Work out the finished part from the listing and answer in its coordinate system (mm). Face numbers are marked on the shaded views. A direction names the side the tool comes from. Coordinates: 2 decimals unless noted, no trailing zeros. Order: outer loops, then holes, each group sorted by start corner. A loop starts at its lowest first (then second) coordinate and runs counter-clockwise, first axis right, second up. Notation, with made-up numbers: M -21.75,51 L 18.25,51 A12 cw 18.25,55 Z; hole C 62,86.25 d10. An arc over 180 degrees is marked long. Write item = value, one per line. Start each with the question number.
Q1. Straight lines are drawn through the part: line 1 along Y through (x, z) = (1.25, 13); line 2 along Z through (x, y) = (0.25, -3); line 3 along X through (y, z) = (-1, 19). For each, find the intervals that lie inside material, in ascending order.
Q2. A tool of negligible diameter and unlimited length cuts with its end or side. For the marked faces 1, 2 and 3, from which of +Z, -Z, +X, -X, +Y, -Y can it reach the whole face along a straight path? Write none if from no direction.
Q3. Find section B-B on x = 2.5. Give the vertices of the cut face in (y, z).
Q4. Find section C-C on z = 11. Give the vertices of the cut face in (x, y).
Q5. Find section A-A on y = 1.5. Give the vertices of the cut face in (x, z), and give its area (3 significant figures).
Q6. Each of these flat-tipped pins is pushed along its axis until it touches: P1, Ø1.5, axis at x = 2.5, z = 14.5, coming from the +Y side; P2, Ø1.2, axis at y = 0, z = 16.5, coming from the +X side; P3, Ø3, axis at y = -1, z = 17.5, coming from the -X side; P4, Ø5, axis at x = 1, y = 1.5, coming from the -Z side. Where does it stop, or does it pass through?
Q7. Find section D-D on y = -3.25. Give the vertices of the cut face in (x, z), and give its area (3 significant figures).
Autodesk Inventor part; units mm, degrees
ref_plane "YZ Plane" through (0, 0, 0) normal (1, 0, 0) x (0, 1, 0)
ref_plane "XZ Plane" through (0, 0, 0) normal (0, 1, 0) x (-1, 0, 0)
ref_plane "XY Plane" through (0, 0, 0) normal (0, 0, 1) x (1, 0, 0)
sketch "Sketch1" plane through (0, 0, 0) normal (0, 0, 1) x (1, 0, 0)
  line L0 (-4.45, 4.45) -> (4.45, 4.45)
  line L1 (4.45, 4.45) -> (4.45, -4.45)
  line L2 (4.45, -4.45) -> (-4.45, -4.45)
  line L3 (-4.45, -4.45) -> (-4.45, 4.45)
  point P0 (0, 0)
  dimension "d0" = 8.9
  dimension "d1" = 8.9
  dimension "d2" = 4.45
  dimension "d3" = 4.45
extrude "Extrusion1" add sketch "Sketch1" along normal blind 10
sketch "Sketch2" plane through (0, 0, 10) normal (0, 0, 1) x (1, 0, 0)
  line L0 (-3, 2) -> (3, 2)
  line L1 (3, 2) -> (3, -2)
  line L2 (3, -2) -> (-3, -2)
  line L3 (-3, -2) -> (-3, 2)
  point P0 (0, 0)
  dimension "d6" = 4
  dimension "d7" = 6
  dimension "d8" = 2
  dimension "d9" = 3
extrude "Extrusion2" add sketch "Sketch2" along normal blind 10
equation "\"d1\" = d0"
properties part number "PulleySocket"
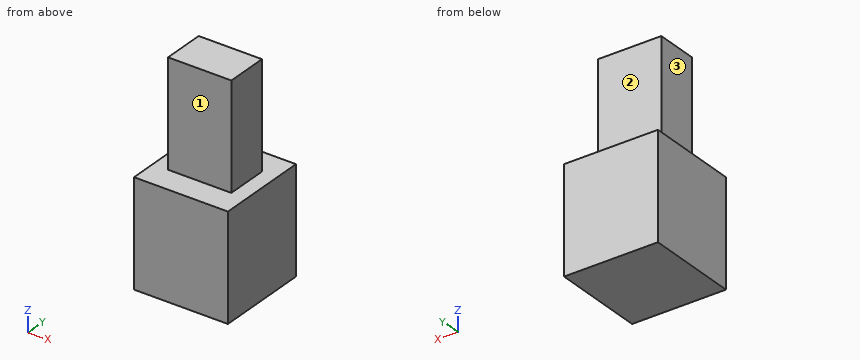
Findings below:
q1.line_1 = -2 to 2
q1.line_2 = 0 to 10
q1.line_3 = -3 to 3
q2.face_1 = +Z, +X, -X, -Y
q2.face_2 = +Z, +X, -X, +Y
q2.face_3 = +Z, -X, +Y, -Y
q3.outline = M -4.45,0 L 4.45,0 L 4.45,10 L 2,10 L 2,20 L -2,20 L -2,10 L -4.45,10 Z
q4.outline = M -3,-2 L 3,-2 L 3,2 L -3,2 Z
q5.outline = M -4.45,0 L 4.45,0 L 4.45,10 L 3,10 L 3,20 L -3,20 L -3,10 L -4.45,10 Z
q5.area = 149 mm^2
q6.P1 = 2
q6.P2 = 3
q6.P3 = -3
q6.P4 = 0
q7.outline = M -4.45,0 L 4.45,0 L 4.45,10 L -4.45,10 Z
q7.area = 89.0 mm^2
